```python
from build123d import *

# Parameters (mm, degrees)
SKETCH_1_W          = 520
SKETCH_1_H          = 420
EXTRUDE_2_DEPTH     = 5
SKETCH_2_R          = 2.5
CUT_EXTRUDE_1_DEPTH = 335.252898267
FILLET_1_R          = 5
CUT_EXTRUDE_2_DEPTH = 10


with BuildPart() as part:
    # 草图1 → 凸台-拉伸2 (new body)
    with BuildSketch(Plane.XY):
        Rectangle(SKETCH_1_W, SKETCH_1_H)
    extrude(amount=EXTRUDE_2_DEPTH)

    # 草图2 → 切除-拉伸1 (cut, through all)
    with BuildSketch(Plane(origin=(0, 0, 0), x_dir=(-1, 0, 0), z_dir=(0, 0, -1))):
        with Locations((-180, 200)):
            Circle(SKETCH_2_R)
        with Locations((-250, 130)):
            Circle(SKETCH_2_R)
        with Locations((-250, -130)):
            Circle(SKETCH_2_R)
        with Locations((-180, -200)):
            Circle(SKETCH_2_R)
        with Locations((180, -200)):
            Circle(SKETCH_2_R)
        with Locations((250, -130)):
            Circle(SKETCH_2_R)
        with Locations((250, 130)):
            Circle(SKETCH_2_R)
        with Locations((180, 200)):
            Circle(SKETCH_2_R)
        Polygon((240, -190), (240, -150), (260, -150), (260, -210), (200, -210), (200, -190), align=None)
        Polygon((240, 190), (200, 190), (200, 210), (260, 210), (260, 150), (240, 150), align=None)
        Polygon((-240, 190), (-240, 150), (-260, 150), (-260, 210), (-200, 210), (-200, 190), align=None)
        Polygon((-240, -190), (-200, -190), (-200, -210), (-260, -210), (-260, -150), (-240, -150), align=None)
    extrude(amount=-CUT_EXTRUDE_1_DEPTH, mode=Mode.SUBTRACT)

    # 圆角1
    fillet_1_edges = [part.edges().sort_by_distance(p)[0] for p in [
        (-240, 150, 2.5),
        (-240, 190, 2.5),
        (-200, 190, 2.5),
        (-200, 210, 2.5),
        (-260, 150, 2.5),
        (-200, -190, 2.5),
        (-240, -190, 2.5),
        (-240, -150, 2.5),
        (-260, -150, 2.5),
        (-200, -210, 2.5),
        (260, -150, 2.5),
        (240, -150, 2.5),
        (240, -190, 2.5),
        (200, -190, 2.5),
        (200, -210, 2.5),
        (200, 210, 2.5),
        (200, 190, 2.5),
        (240, 190, 2.5),
        (240, 150, 2.5),
        (260, 150, 2.5),
    ]]
    fillet(fillet_1_edges, radius=FILLET_1_R)

    # 草图3 → 切除-拉伸2 (cut)
    with BuildSketch(Plane.XY.offset(5)):
        with BuildLine():
            Line((-210, -95), (-60, -95))
            ThreePointArc((-60, -95), (-57.5, -92.5), (-60, -90))
            Line((-60, -90), (-210, -90))
            ThreePointArc((-210, -90), (-212.5, -92.5), (-210, -95))
        make_face()
        with BuildLine():
            Line((-210, -160), (-60, -160))
            ThreePointArc((-60, -160), (-57.5, -157.5), (-60, -155))
            Line((-60, -155), (-210, -155))
            ThreePointArc((-210, -155), (-212.5, -157.5), (-210, -160))
        make_face()
        with BuildLine():
            Line((60, -160), (210, -160))
            ThreePointArc((210, -160), (212.5, -157.5), (210, -155))
            Line((210, -155), (60, -155))
            ThreePointArc((60, -155), (57.5, -157.5), (60, -160))
        make_face()
        with BuildLine():
            Line((60, -95), (210, -95))
            ThreePointArc((210, -95), (212.5, -92.5), (210, -90))
            Line((210, -90), (60, -90))
            ThreePointArc((60, -90), (57.5, -92.5), (60, -95))
        make_face()
    extrude(amount=-CUT_EXTRUDE_2_DEPTH, mode=Mode.SUBTRACT)


solid = part.part
```
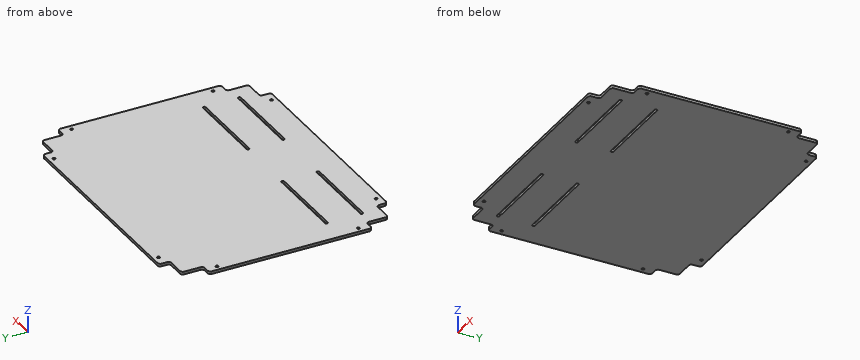
The listing builds one solid part. Answer for the finished solid, in the listing's coordinates (mm). Give positions to 0.01 mm unless a question says otherwise; leave off trailing zeros. Order: outer loops, then holes, each group sorted by start corner. A loop starts at its lowest first (then second) coordinate and runs counter-clockwise, first axis right, second up. Notation, with made-up numbers: (22.25, 67) - (71.25, 67) arc R24 cw to (71.25, 99) - close; hole circle Ø11 at (73, 45). An arc over 180 degrees is marked (long way). Answer in a Markdown table with one row per item. Add a question column.
Q1. The part is cut by section B-B (z = 4.1). Give the number of separate pieces and of enclosed holes in the cut face, then the cut area to 3 significant figures.
Q2. Given P1, Ø1.5, axis at y = 198.5, z = 3.5, coming from the -X side; P2, Ø2.5, axis at x = -223.5, z = 3, coming from the -Y side; P3, Ø4.5, axis at x = 180, y = 200, coming from the +Z side; P4, Ø2.5, axis at x = -250.5, z = 2, coming from the -Y side, each flat-ended and moving along its own axis, determine where each tip first touches the part or whether it passes through.
Q3. Find the intervals of material crossed by line 1 along Y through (x, z) = (209.5, 4.15); line 2 along Y through (x, z) = (-180, 1.6); line 3 along Y through (x, z) = (-150, 2.9), in increasing order. Write a range as [from, to].
Q4. The part is cut by section A-A (x = -131.5). Determine the outline of the cut face in (y, z).
Determined:
| question | item | result |
|---|---|---|
| 1 | separate pieces | 1 |
| 1 | enclosed holes | 12 |
| 1 | area | 207,000 mm² |
| 2 | P1 | stops at x = -200 |
| 2 | P2 | stops at y = -190 |
| 2 | P3 | passes through |
| 2 | P4 | stops at y = -150 |
| 3 | line 1 | y = [-190, -160], [-155, -95], [-90, 190] |
| 3 | line 2 | y = [-210, -202.5], [-197.5, -160], [-155, -95], [-90, 197.5], [202.5, 210] |
| 3 | line 3 | y = [-210, -160], [-155, -95], [-90, 210] |
| 4 | outline | (-210, 0) - (-160, 0) - (-160, 5) - (-210, 5) - close; (-155, 0) - (-95, 0) - (-95, 5) - (-155, 5) - close; (-90, 0) - (210, 0) - (210, 5) - (-90, 5) - close |
